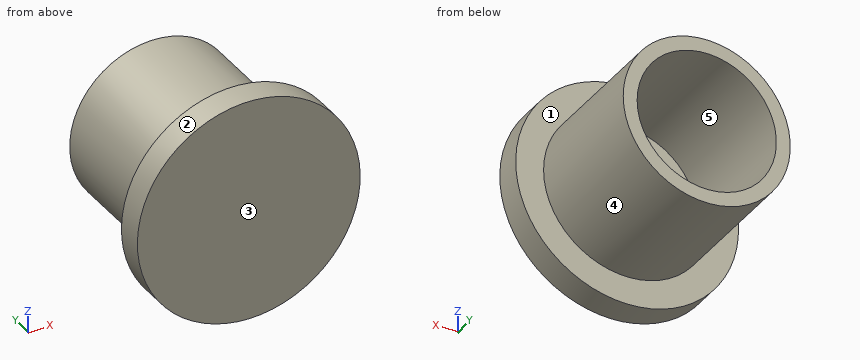
```python
from build123d import *

# Parameters (mm, degrees)
ESQUISSE1_R    = 6
ESQUISSE1_R_2  = 5
CYLINDRE_DEPTH = 10
ESQUISSE2_R    = 8
BASE_DEPTH     = 2


with BuildPart() as part:
    # Esquisse1 → Cylindre (new body)
    with BuildSketch(Plane(origin=(0, 0, 0), x_dir=(1, 0, 0), z_dir=(0, 1, 0))):
        Circle(ESQUISSE1_R)
        Circle(ESQUISSE1_R_2, mode=Mode.SUBTRACT)
    extrude(amount=CYLINDRE_DEPTH)

    # Esquisse2 → Base (add)
    with BuildSketch(Plane.XZ):
        with Locations(Location((0, 0, 0), (0, 0, 270))):
            Circle(ESQUISSE2_R)
    extrude(amount=BASE_DEPTH)


solid = part.part
```
Input: part model. Units: mm. Frame: model coordinates. Face numbers are marked on the shaded views. A direction names the side the tool comes from. Round coordinates to 2 decimals unless told otherwise and drop trailing zeros. Loops run counter-clockwise (first coordinate to the right, second up) from the corner with the lowest first, then second, coordinate; pieces in that order, holes last. Notation, with made-up numbers: (39, 72) -> (90, 72) arc R19 ccw to (90, 109) -> close; hole circle Ø10 at (-23, -30). An arc over 180 degrees is marked (long way). One line per item, written item: value.
(1) Section D-D (z = 5.25). Return the cut outline in (x, y).
Geometry check:
outline: (-6.04, -2) -> (6.04, -2) -> (6.04, 0) -> (2.9, 0) -> (2.9, 10) -> (-2.9, 10) -> (-2.9, 0) -> (-6.04, 0) -> close
(2) Set-up query: the marked faces 1 and 2. Return all of +Z, -Z, +X, -X, +Y, -Y with unobstructed straight access to the full face (end or side cutting, diameter ignored); none if empty.
Geometry check:
face 1: +Y
face 2: +Y, -Y
(3) Material intervals for line 1 (X direction, y = 6, z = 0); line 2 (Y direction, x = -0.5, z = 4.75), sorted ascending. Write a range as [from, to].
Geometry check:
line 1: [-6, -5], [5, 6]
line 2: [-2, 0]
(4) Pin query (flat end, axial travel): pin 1 (2 mm diameter, centred on y = 6, z = 0, fed in from -X); pin 2 (1 mm diameter, centred on y = 7.5, z = 2, fed in from -X); pin 3 (1.5 mm diameter, centred on x = -1, z = -0.5, fed in from +Y). Return the tip coordinate at first contact, or that it passes through.
Geometry check:
pin 1: x = -6
pin 2: x = -5.81
pin 3: y = 0
(5) Mould query, pull axis Z, two halves, no side actions, for the marked faces 3, 4 and 5. Classes: pulls with the +Z half, pulls with the -Z half, needs draft (parallel to the pull), parting line crosses it, or undercut.
Geometry check:
face 3: needs draft
face 4: parting line crosses it
face 5: undercut
(6) Section A-A (z = 0). Return the cut outline in (x, y), plus the area to 3 significant figures.
Geometry check:
outline: (-8, -2) -> (8, -2) -> (8, 0) -> (6, 0) -> (6, 10) -> (5, 10) -> (5, 0) -> (-5, 0) -> (-5, 10) -> (-6, 10) -> (-6, 0) -> (-8, 0) -> close
area: 52.0 mm2
(7) Section C-C (y = 3). Return the cut outline in (x, z), plus the area to 3 significant figures.
Geometry check:
outline: circle Ø12 at (0, 0); hole circle Ø10 at (0, 0)
area: 34.6 mm2
(8) Section B-B (x = 0). Return the cut outline in (y, z), plus the area to 3 significant figures.
Geometry check:
outline: (-2, -8) -> (0, -8) -> (0, -6) -> (10, -6) -> (10, -5) -> (0, -5) -> (0, 5) -> (10, 5) -> (10, 6) -> (0, 6) -> (0, 8) -> (-2, 8) -> close
area: 52.0 mm2
